```python
from build123d import *

# Parameters (mm, degrees)
F0_R     = 16.25
F0_R_2   = 14.25
F0_R_3   = 12.25
F1_DEPTH = 2
F2_DEPTH = 11
F3_SIZE  = 1
F4_R     = 0.5


with BuildPart() as f1:
    # F0 (on Front) → F1 (new body)
    with BuildSketch(Plane.XZ):
        Circle(F0_R)
        Circle(F0_R_2, mode=Mode.SUBTRACT)
        Circle(F0_R_2)
        Circle(F0_R_3, mode=Mode.SUBTRACT)
    extrude(amount=F1_DEPTH)

    # F0 (on Front) → F2 (join)
    with BuildSketch(Plane.XZ):
        Circle(F0_R)
        Circle(F0_R_2, mode=Mode.SUBTRACT)
    extrude(amount=F2_DEPTH)

    # F3
    f3_edges = [f1.edges().sort_by_distance(p)[0] for p in [
        (-14.25, -11, 0),
        (-12.25, -2, 0),
    ]]
    chamfer(f3_edges, length=F3_SIZE)

    # F4
    f4_edges = [f1.edges().sort_by_distance(p)[0] for p in [
        (-16.25, 0, 0),
        (16.25, -5.5, 0),
        (-16.25, -11, 0),
        (-12.25, 0, 0),
        (-14.25, -10, 0),
        (-13.25, -2, 0),
    ]]
    fillet(f4_edges, radius=F4_R)


solid = f1.part
```
Geometry: final body of the model. Coordinates: model frame, mm. A direction names the side the tool comes from. Coordinates: 2 decimals unless noted, no trailing zeros. Order: outer loops, then holes, each group sorted by start corner. A loop starts at its lowest first (then second) coordinate and runs counter-clockwise, first axis right, second up. Notation, with made-up numbers: (-33, 27) -> (3, 27) arc R29 ccw to (3, 64) -> close; hole circle Ø9 at (54.25, -6). An arc over 180 degrees is marked (long way). Write each question's results on one line, items separated by ' | '. Start each with the question number.
1) First-contact query: pin 1 (17 mm diameter, centred on x = 0, z = 0, fed in from -Y); pin 2 (3 mm diameter, centred on x = -3, y = -7, fed in from +Z); pin 3 (1 mm diameter, centred on x = 3.5, y = -1.5, fed in from -Z); pin 4 (3 mm diameter, centred on y = -8.5, z = -6, fed in from -X). Flat tips, straight axial feed; report the tip coordinate or a pass-through.
2) Set-up query: faces 1 (the cylindrical face through (13.163, -5.842, -5.458)), 2 (the flat face through (13, 0, 0)). Return all of +Z, -Z, +X, -X, +Y, -Y with unobstructed straight access to the full face (end or side cutting, diameter ignored); none if empty.
3) Material intervals for line 1 along Z through (x, y) = (0, -5.25); line 2 along Z through (x, y) = (0, -0.7); line 3 along X through (y, z) = (-9.5, -0.5), sorted ascending.
4) Cut plane A-A, the plane y = -8.25. Output: boundary loops of the cut face in (x, z).
Checks:
1) pin 1: through | pin 2: z = 16.18 | pin 3: z = -15.97 | pin 4: x = -15.61
2) face 1: -Y | face 2: +Z, -Z, +X, -X, +Y
3) line 1: -16.25 to -14.25, 14.25 to 16.25 | line 2: -16.25 to -12.25, 12.25 to 16.25 | line 3: -16.24 to -14.24, 14.24 to 16.24
4) outline: circle Ø32.5 at (0, 0); hole circle Ø28.5 at (0, 0)
